Design review of the part shown in the three views and the two pictorial views. Dimensions are in mm from the part's minimum x, y and z. Give positions to 0.01 mm unless a question says otherwise; leave off trailing zeros. Loops run counter-clockwise (first coordinate to the right, second up) from the corner with the lowest first, then second, coordinate; pieces in that order, holes last. Notation, with made-up numbers: (4, 30) -> (11, 30) arc R10 ccw to (11, 37) -> close; hole circle Ø1 at (-35.5, -39.5). An arc over 180 degrees is marked (long way). One line per question, with ' | ' between items. Start each with the question number.
(1) Consider section B-B (z = 26). Write out the cut boundary in (x, y), and give its area (3 significant figures).
(2) Insertion check: P1, Ø0.9, axis at x = 2, y = 1.5, coming from the -Z side; P2, Ø3, axis at x = 5.5, z = 16, coming from the -Y side; P3, Ø1.5, axis at x = 10.5, y = 1.5, coming from the -Z side; P4, Ø0.9, axis at y = 1, z = 1.5, coming from the +X side. Each pin has a flat end and moves straight along its axis. Give the tip position at first contact, or say it passes through.
(3) Wall thickness on probe 1 along Z at (x, y) = (12.75, 1.2); probe 2 along Z at (x, y) = (4.25, 0.8); probe 3 along X at (y, z) = (2.5, 15.5): over which ranges is each line inside the solid? List them lowest first.
(4) Consider section D-D (x = 2). Write out the cut boundary in (y, z), and give its area (3 significant figures).
(5) Consider section C-C (y = 0.65). Write out the cut boundary in (x, z), and give its area (3 significant figures).
(6) Consider section A-A (x = 7.75). Write out the cut boundary in (y, z), and give its area (3 significant figures).
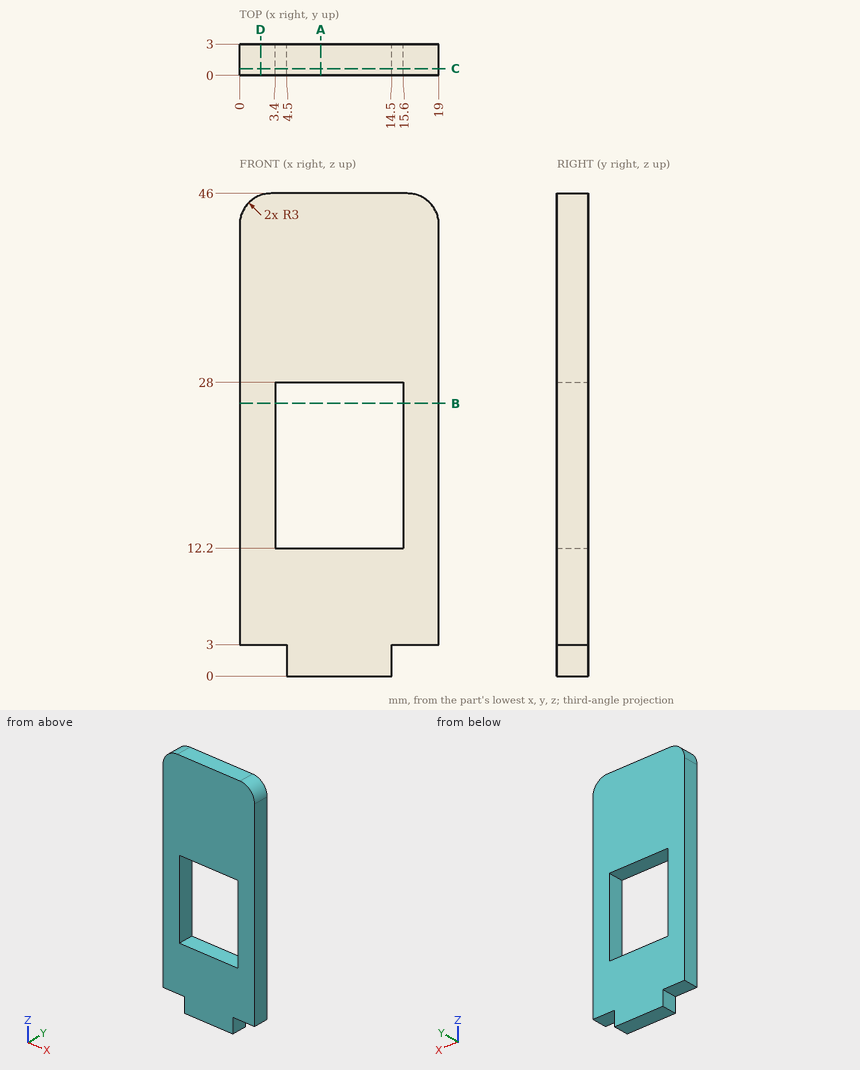
A:
1) outline: (0, 0) -> (3.4, 0) -> (3.4, 3) -> (0, 3) -> close; (15.6, 0) -> (19, 0) -> (19, 3) -> (15.6, 3) -> close | area: 20.4 mm^2
2) P1: stops at z = 3 | P2: passes through | P3: stops at z = 0 | P4: stops at x = 14.5
3) probe 1: z = 0 to 12.2, 28 to 46 | probe 2: z = 3 to 12.2, 28 to 46 | probe 3: x = 0 to 3.4, 15.6 to 19
4) outline: (0, 3) -> (3, 3) -> (3, 45.83) -> (0, 45.83) -> close | area: 128 mm^2
5) outline: (0, 3) -> (4.5, 3) -> (4.5, 0) -> (14.5, 0) -> (14.5, 3) -> (19, 3) -> (19, 43) arc R3 ccw to (16, 46) -> (3, 46) arc R3 ccw to (0, 43) -> close; hole (3.4, 12.2) -> (15.6, 12.2) -> (15.6, 28) -> (3.4, 28) -> close | area: 650 mm^2
6) outline: (0, 0) -> (3, 0) -> (3, 12.2) -> (0, 12.2) -> close; (0, 28) -> (3, 28) -> (3, 46) -> (0, 46) -> close | area: 90.6 mm^2
